Can you work these out from the drawing? Everything is in mm from the part's minimum corner. Round coordinates to 2 decimals unless told otherwise and drop trailing zeros. Loops run counter-clockwise (first coordinate to the right, second up) from the corner with the lowest first, then second, coordinate; pieces in that order, holes last. Notation, with made-up numbers: (64, 77) -> (78, 77) arc R18 ccw to (78, 90) -> close; hole circle Ø6 at (11, 2). An arc over 180 degrees is marked (long way). One line per item, written item: value.
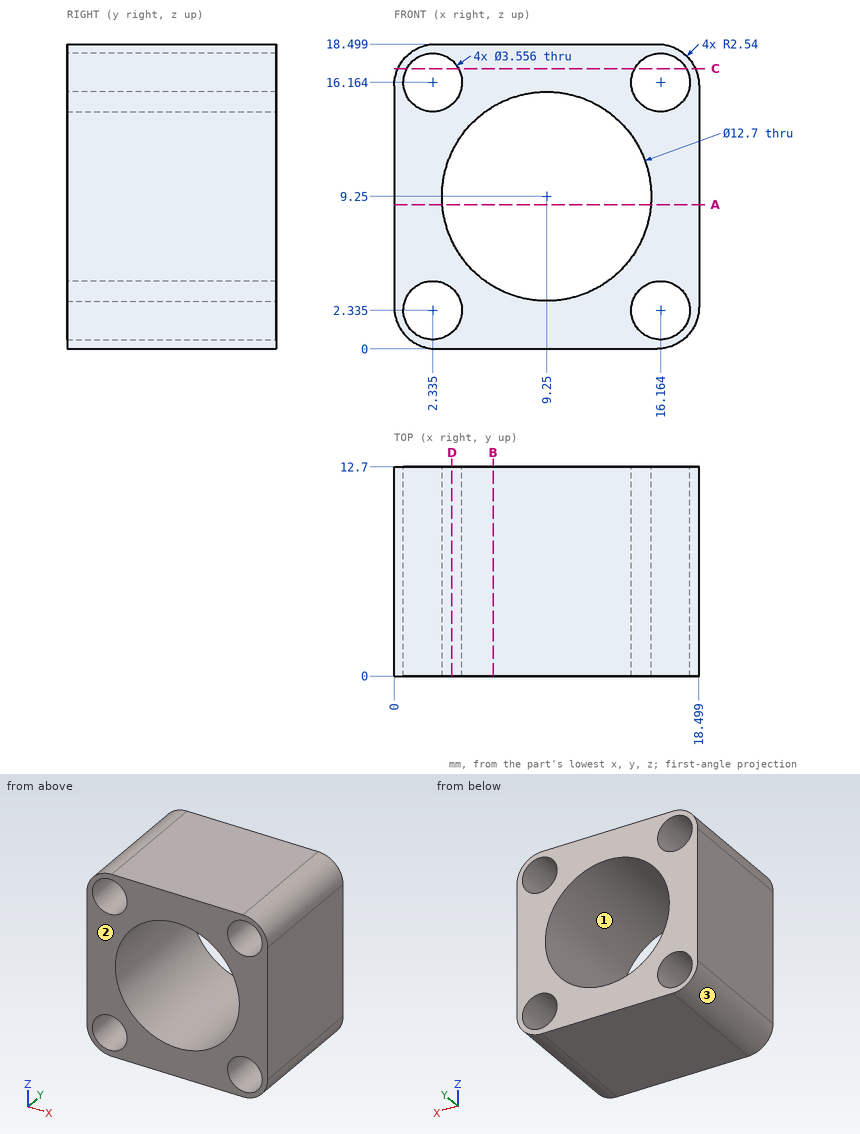
(1) Imagine slicing it at A-A on z = 8.75. Write out the boundary of the cut face in (x, y).
Results below:
outline: (0, 0) -> (2.92, 0) -> (2.92, 12.7) -> (0, 12.7) -> close; (15.58, 0) -> (18.5, 0) -> (18.5, 12.7) -> (15.58, 12.7) -> close
(2) We'd pull the mould along Z, two halves only. Please class the marked faces 1, 2 and 3: +Z half, -Z half, draft (parallel to the pull), parting line (faces both ways), or undercut.
Results below:
face 1: undercut
face 2: draft
face 3: -Z half
(3) Imagine slicing it at D-D on x = 3.5. Write out the boundary of the cut face in (y, z) (1 decimal).
Results below:
outline: (0, 0) -> (12.7, 0) -> (12.7, 1) -> (0, 1) -> close; (0, 3.7) -> (12.7, 3.7) -> (12.7, 6.6) -> (0, 6.6) -> close; (0, 11.9) -> (12.7, 11.9) -> (12.7, 14.8) -> (0, 14.8) -> close; (0, 17.5) -> (12.7, 17.5) -> (12.7, 18.5) -> (0, 18.5) -> close
(4) Imagine slicing it at B-B on x = 6. Write out the boundary of the cut face in (y, z) (1 decimal).
Results below:
outline: (0, 0) -> (12.7, 0) -> (12.7, 3.8) -> (0, 3.8) -> close; (0, 14.7) -> (12.7, 14.7) -> (12.7, 18.5) -> (0, 18.5) -> close
(5) Please list where these lines run through material, in increasing order: L1, parallel to Z at x = 9, y = 8.75 (1 decimal); L2, parallel to X at y = 5.5, z = 15 (1 decimal).
Results below:
L1: z = 0 to 2.9, 15.6 to 18.5
L2: x = 0 to 1, 3.7 to 6.6, 11.9 to 14.8, 17.5 to 18.5
(6) Imagine slicing it at C-C on z = 17. Write out the boundary of the cut face in (x, y) (1 decimal).
Results below:
outline: (0.2, 0) -> (0.8, 0) -> (0.8, 12.7) -> (0.2, 12.7) -> close; (3.9, 0) -> (14.6, 0) -> (14.6, 12.7) -> (3.9, 12.7) -> close; (17.7, 0) -> (18.3, 0) -> (18.3, 12.7) -> (17.7, 12.7) -> close
